Verification items for the finished model (mm, model axes). Round coordinates to 2 decimals unless told otherwise and drop trailing zeros. Use one line per item in the form item = value. Start each with the question number.
Item 1: Cross-section at A-A on y = 5.35. Count the separate pieces of the cut face and the enclosed holes in it, then the cut area to 3 significant figures.
Item 2: Thickness scan on probe 1 along X at (y, z) = (4.15, 169); probe 2 along X at (y, z) = (4.55, 49); probe 3 along Z at (x, y) = (148.5, 4.9). Record the ranges inside material, lowest first. Write a range as [from, to].
Item 3: Go/stop test with a flat-tipped pin: pin 1 Ø2.5 at (x, z) = (325.47, 71) entering from -Y. Record where the tip stops, or that it passes through.
from build123d import *

# Parameters (mm, degrees)
SKETCH_1_W          = 350
SKETCH_1_H          = 3
EXTRUDE_1_DEPTH     = 490
SKETCH_2_R          = 2.6
SKETCH_2_R_2        = 2.25
SKETCH_2_R_3        = 2.1
SKETCH_2_W          = 60
SKETCH_2_H          = 380
CUT_EXTRUDE_1_DEPTH = 50


with BuildPart() as part:
    # 草图1 → 凸台-拉伸1 (new body)
    with BuildSketch(Plane.XY):
        with Locations((156.473684211, 4.735473664)):
            Rectangle(SKETCH_1_W, SKETCH_1_H)
    extrude(amount=EXTRUDE_1_DEPTH)

    # 草图2 → 切除-拉伸1 (cut)
    with BuildSketch(Plane(origin=(0, 6.235473664, 0), x_dir=(1, 0, 0), z_dir=(0, 1, 0))):
        with Locations((-11.026315789, -48.5)):
            Circle(SKETCH_2_R)
        with Locations((83.973684211, -48.5)):
            Circle(SKETCH_2_R)
        with Locations((-11.026315789, -443.5)):
            Circle(SKETCH_2_R)
        with Locations((83.973684211, -443.5)):
            Circle(SKETCH_2_R)
        with Locations((310.473684211, -159)):
            Circle(SKETCH_2_R_2)
        with Locations((325.473684211, -159)):
            Circle(SKETCH_2_R_2)
        with Locations((325.473684211, -169)):
            Circle(SKETCH_2_R_2)
        with Locations((310.473684211, -169)):
            Circle(SKETCH_2_R_2)
        with Locations((310.473684211, -431)):
            Circle(SKETCH_2_R_2)
        with Locations((325.473684211, -431)):
            Circle(SKETCH_2_R_2)
        with Locations((325.473684211, -421)):
            Circle(SKETCH_2_R_2)
        with Locations((310.473684211, -421)):
            Circle(SKETCH_2_R_2)
        with Locations((325.473684211, -149)):
            Circle(SKETCH_2_R_2)
        with Locations((310.473684211, -149)):
            Circle(SKETCH_2_R_2)
        with Locations((310.473684211, -139)):
            Circle(SKETCH_2_R_2)
        with Locations((325.473684211, -139)):
            Circle(SKETCH_2_R_2)
        with Locations((310.473684211, -71)):
            Circle(SKETCH_2_R_2)
        with Locations((310.473684211, -61)):
            Circle(SKETCH_2_R_2)
        with Locations((325.473684211, -61)):
            Circle(SKETCH_2_R_2)
        with Locations((325.473684211, -71)):
            Circle(SKETCH_2_R_2)
        with Locations((281.473684211, -6)):
            Circle(SKETCH_2_R_2)
        with Locations((253.473684211, -6)):
            Circle(SKETCH_2_R_2)
        with Locations((31.473684211, -6)):
            Circle(SKETCH_2_R_2)
        with Locations((59.473684211, -6)):
            Circle(SKETCH_2_R_2)
        with Locations((266.473684211, -24)):
            Circle(SKETCH_2_R_3)
        with Locations((266.473684211, -49)):
            Circle(SKETCH_2_R_3)
        with Locations((266.473684211, -443)):
            Circle(SKETCH_2_R_3)
        with Locations((256.473684211, -443)):
            Circle(SKETCH_2_R_3)
        with Locations((11.473684211, -246)):
            Rectangle(SKETCH_2_W, SKETCH_2_H)
        with BuildLine():
            Line((274.223684211, -472.5), (274.223684211, -477.5))
            ThreePointArc((274.223684211, -477.5), (276.473684211, -479.75), (278.723684211, -477.5))
            Line((278.723684211, -477.5), (278.723684211, -472.5))
            ThreePointArc((278.723684211, -472.5), (276.473684211, -470.25), (274.223684211, -472.5))
        make_face()
        with BuildLine():
            Line((146.223684211, -472.5), (146.223684211, -477.5))
            ThreePointArc((146.223684211, -477.5), (148.473684211, -479.75), (150.723684211, -477.5))
            Line((150.723684211, -477.5), (150.723684211, -472.5))
            ThreePointArc((150.723684211, -472.5), (148.473684211, -470.25), (146.223684211, -472.5))
        make_face()
        with BuildLine():
            Line((18.223684211, -472.5), (18.223684211, -477.5))
            ThreePointArc((18.223684211, -477.5), (20.473684211, -479.75), (22.723684211, -477.5))
            Line((22.723684211, -477.5), (22.723684211, -472.5))
            ThreePointArc((22.723684211, -472.5), (20.473684211, -470.25), (18.223684211, -472.5))
        make_face()
    extrude(amount=-CUT_EXTRUDE_1_DEPTH, mode=Mode.SUBTRACT)


solid = part.part
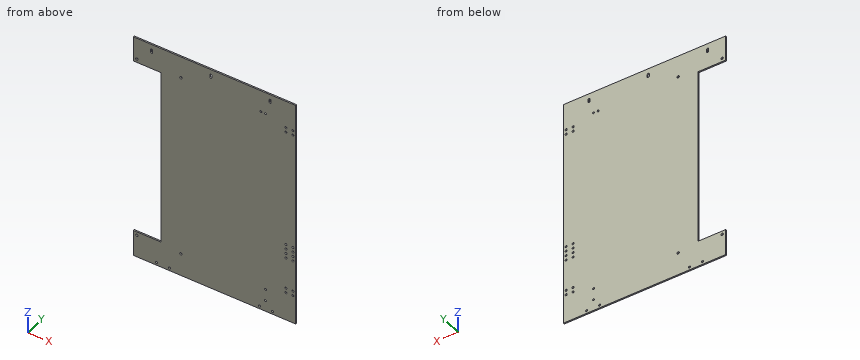
Output values:
q1.separate_pieces = 1
q1.enclosed_holes = 31
q1.area = 148,000 mm2
q2.probe_1 = [41.47, 308.22], [312.72, 323.22], [327.72, 331.47]
q2.probe_2 = [-18.53, -13.58], [-8.47, 81.42], [86.53, 264.37], [268.57, 331.47]
q2.probe_3 = [0, 470.25], [479.75, 490]
q3.pin_1 = through
